Check sheet for the drawn part. Datum: minimum x, y, z corner. Units: mm. A direction names the side the tool comes from. Round coordinates to 2 decimals unless told otherwise and drop trailing zeros. Write each loop counter-clockwise with the first axis right and the second up, starting at its lowest first coordinate (ties: lowest second). Pieces come first, ordered by that corner, then holes.
Item 1: Go/stop test with a flat-tipped pin: pin 1 Ø4 at (x, z) = (55.795, 21.551) entering from -Y. Record where the tip stops, or that it passes through.
Item 2: Cross-section at D-D on z = 21.5. Enter the section's corners in (x, y), plus the area to 3 significant figures.
Item 3: Cross-section at B-B on x = 45. Enter the section's corners in (y, z).
Item 4: Release check for a two-part mould opening along Z. For the marked faces 1, 2 and 3 record: +Z half, -Z half, draft (parallel to the pull), parting line (faces both ways), or undercut.
Item 5: Tool access check on the marked faces 4 and 5. Record the directions out of +Z, -Z, +X, -X, +Y, -Y that give a thin tool (end or side, any length) a straight path to the whole face; none if there is none.
Item 6: Cross-section at A-A on x = 15. Enter the section's corners in (y, z), plus the area to 3 significant figures.
Item 7: Material ranges on line 1 (Z direction, x = 32.5, y = 2.75); line 2 (X direction, y = 7.55, z = 4) (3 decimals); line 3 (Z direction, x = 34.5, y = 7.25), recorded low to high.
Item 8: Cross-section at C-C on y = 5.75. Enter the section's corners in (x, z), plus the area to 3 significant figures.
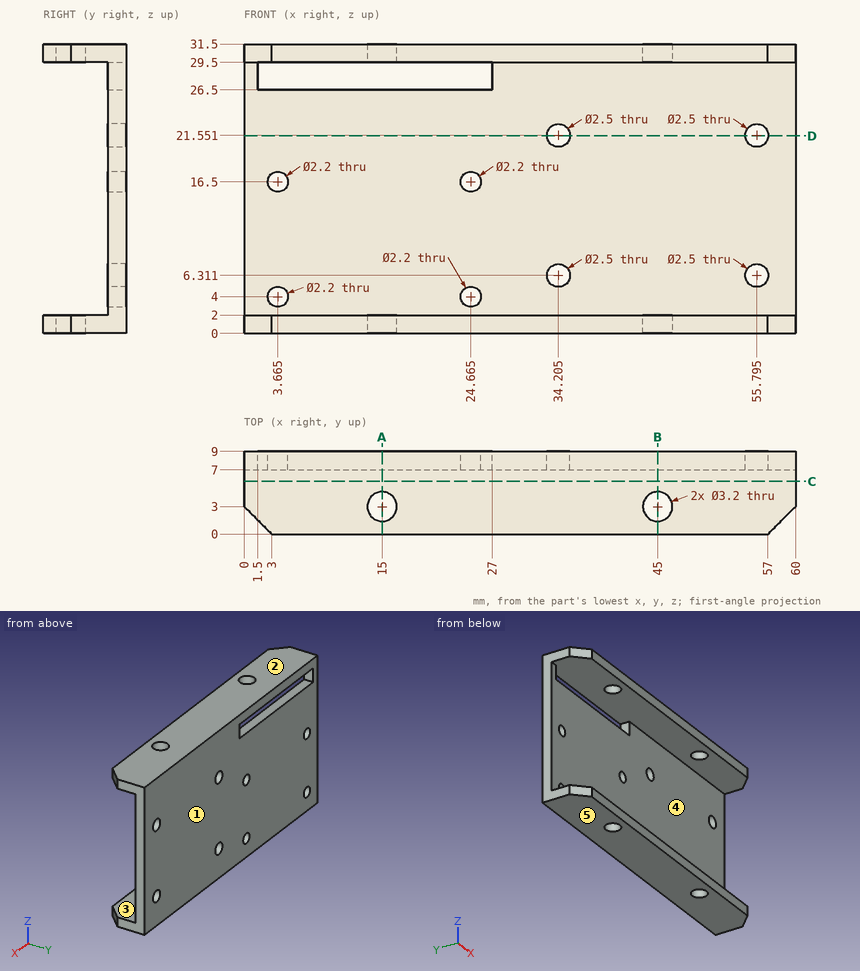
Response values:
1. pin 1: stops at y = 7
2. outline: (0, 7) - (32.96, 7) - (32.96, 9) - (0, 9) - close; (35.45, 7) - (54.55, 7) - (54.55, 9) - (35.45, 9) - close; (57.04, 7) - (60, 7) - (60, 9) - (57.04, 9) - close
2. area: 110 mm2
3. outline: (0, 0) - (1.4, 0) - (1.4, 2) - (0, 2) - close; (0, 29.5) - (1.4, 29.5) - (1.4, 31.5) - (0, 31.5) - close; (4.6, 0) - (9, 0) - (9, 31.5) - (4.6, 31.5) - (4.6, 29.5) - (7, 29.5) - (7, 2) - (4.6, 2) - close
4. face 1: draft
4. face 2: +Z half
4. face 3: undercut
5. face 4: +X, -X, -Y
5. face 5: -Z, +X, -X, +Y, -Y
6. outline: (0, 0) - (1.4, 0) - (1.4, 2) - (0, 2) - close; (0, 29.5) - (1.4, 29.5) - (1.4, 31.5) - (0, 31.5) - close; (4.6, 0) - (9, 0) - (9, 26.5) - (7, 26.5) - (7, 2) - (4.6, 2) - close; (4.6, 29.5) - (9, 29.5) - (9, 31.5) - (4.6, 31.5) - close
6. area: 72.2 mm2
7. line 1: z = 0 to 2, 29.5 to 31.5
7. line 2: x = 0 to 2.565, 4.765 to 23.565, 25.765 to 60
7. line 3: z = 0 to 5.1, 7.53 to 20.34, 22.77 to 31.5
8. outline: (0, 0) - (60, 0) - (60, 2) - (0, 2) - close; (0, 29.5) - (60, 29.5) - (60, 31.5) - (0, 31.5) - close
8. area: 240 mm2
